```python
from build123d import *

# Parameters (mm, degrees)
F0_W     = 63.5
F0_H     = 127
F1_DEPTH = 6.35
F2_W     = 63.5
F2_H     = 6.35
F3_DEPTH = 50.8
F5_DEPTH = 25.4


with BuildPart() as f1:
    # F0 (on Front) → F1 (new body)
    with BuildSketch(Plane.XZ):
        with Locations((-105.7790880203, 53.5060482323)):
            Rectangle(F0_W, F0_H)
    extrude(amount=F1_DEPTH)

    # F2 (on face) → F3 (join)
    with BuildSketch(Plane(origin=(0, 0, 0), x_dir=(-1, 0, 0), z_dir=(0, 1, 0))):
        with Locations((105.7790880203, -6.8189517677)):
            Rectangle(F2_W, F2_H)
    extrude(amount=F3_DEPTH)

    # F4 (on face) → F5 (cut)
    with BuildSketch(Plane.XZ.offset(6.35)):
        with BuildLine():
            Line((-105.7790880203, 77.6360482323), (-105.7790880203, 92.8760482323))
            ThreePointArc((-105.7790880203, 92.8760482323), (-113.3990880203, 85.2560482323), (-105.7790880203, 77.6360482323))
        make_face()
        with BuildLine():
            ThreePointArc((-98.1590880203, 85.2560482323), (-100.3909343477, 90.644201905), (-105.7790880203, 92.8760482323))
            Line((-105.7790880203, 92.8760482323), (-105.7790880203, 77.6360482323))
            ThreePointArc((-105.7790880203, 77.6360482323), (-100.3909343477, 79.8678945597), (-98.1590880203, 85.2560482323))
        make_face()
    extrude(amount=-F5_DEPTH, mode=Mode.SUBTRACT)


solid = f1.part
```
Geometry check sheet. Reference: the model listing, model coordinates, mm. A direction names the side the tool comes from. Give positions to 0.01 mm unless a question says otherwise; leave off trailing zeros. Order: outer loops, then holes, each group sorted by start corner. A loop starts at its lowest first (then second) coordinate and runs counter-clockwise, first axis right, second up. Notation, with made-up numbers: (46.25, 66.25) - (71.25, 66.25) arc R20 ccw to (71.25, 95.25) - close; hole circle Ø5 at (-22, 60.5). An arc over 180 degrees is marked (long way). Answer in a Markdown table with one row per item. Add a question column.
Q1. Gauge pin test, flat ends, axial feed: pin 1 (12 mm diameter, centred on x = -131, z = 30, fed in from +Y); pin 2 (6 mm diameter, centred on x = -110.5, y = 21.5, fed in from +Z); pin 3 (1.5 mm diameter, centred on y = 2.5, z = 11, fed in from -X). Record the tip position at first contact, or that the pin passes through.
Q2. Tool access check on faces 1 (the flat face through (-137.529, -1, 39)), 2 (the flat face through (-106, 0, 58)). Record the directions out of +Z, -Z, +X, -X, +Y, -Y that give a thin tool (end or side, any length) a straight path to the whole face; none if there is none.
Q3. Material ranges on probe 1 along Y at (x, z) = (-104.5, 75); probe 2 along Z at (x, y) = (-96, 8), recorded low to high. Write a range as from..to.
Q4. Cross-section at A-A, the plane x = -102. Enter the section's corners in (y, z).
Q5. Cross-section at C-C, the plane z = 60. Enter the section's corners in (x, y), then the cut area to 3 significant figures.
Q6. Cross-section at B-B, the plane z = 82. Enter the section's corners in (x, y), then the cut area to 3 significant figures.
Q7. Cross-section at D-D, the plane x = -121. Enter the section's corners in (y, z).
Check values:
| question | item | result |
|---|---|---|
| 1 | pin 1 | stops at y = 0 |
| 1 | pin 2 | stops at z = -3.64 |
| 1 | pin 3 | passes through |
| 2 | face 1 | +Z, -Z, -X, +Y, -Y |
| 2 | face 2 | +Z, +X, -X, +Y |
| 3 | probe 1 | y = -6.35..0 |
| 3 | probe 2 | z = -9.99..-3.64 |
| 4 | outline | (-6.35, -9.99) - (50.8, -9.99) - (50.8, -3.64) - (0, -3.64) - (0, 78.64) - (-6.35, 78.64) - close; (-6.35, 91.87) - (0, 91.87) - (0, 117.01) - (-6.35, 117.01) - close |
| 5 | outline | (-137.53, -6.35) - (-74.03, -6.35) - (-74.03, 0) - (-137.53, 0) - close |
| 5 | area | 403 mm^2 |
| 6 | outline | (-137.53, -6.35) - (-112.67, -6.35) - (-112.67, 0) - (-137.53, 0) - close; (-98.89, -6.35) - (-74.03, -6.35) - (-74.03, 0) - (-98.89, 0) - close |
| 6 | area | 316 mm^2 |
| 7 | outline | (-6.35, -9.99) - (50.8, -9.99) - (50.8, -3.64) - (0, -3.64) - (0, 117.01) - (-6.35, 117.01) - close |
